Autodesk Inventor part; units mm, degrees
ref_plane "YZ Plane" through (0, 0, 0) normal (1, 0, 0) x (0, 1, 0)
ref_plane "XZ Plane" through (0, 0, 0) normal (0, 1, 0) x (-1, 0, 0)
ref_plane "XY Plane" through (0, 0, 0) normal (0, 0, 1) x (1, 0, 0)
sketch "Sketch1" plane through (0, 0, 0) normal (0, 1, 0) x (-1, 0, 0)
  line L0 (0, 0) -> (38.1, 0)
  line L1 (38.1, 0) -> (38.1, -50.8)
  line L2 (38.1, -50.8) -> (0, -50.8)
  line L3 (0, -50.8) -> (0, 0)
  line L4 (38.1, -50.8) -> (33.02, -50.8)
  line L5 (33.02, -50.8) -> (33.02, 0)
  line L6 (33.02, 0) -> (38.1, 0)
  line L7 (38.1, 0) -> (38.1, -50.8)
  line L8 (0, -50.8) -> (5.08, -50.8)
  line L9 (5.08, -50.8) -> (5.08, 0)
  line L10 (5.08, 0) -> (0, 0)
  line L11 (0, 0) -> (0, -50.8)
  dimension "d0" = 38.1
  dimension "d1" = 50.8
  dimension "d2" = 5.08
  dimension "d3" = 5.08
extrude "Extrusion1" add sketch "Sketch1" along normal blind 25.4 contours L0 L9 L2 L3 | L0 L1 L2 L5
extrude "Extrusion2" add sketch "Sketch1" against normal blind 13.97
sketch "Sketch2" plane through (0, 25.4, 0) normal (1, 0, 0) x (0, 0, -1)
  line L0 (50.8, 0) -> (0, 0)
  line L1 (25.4, 0) -> (25.4, -12.7)
  point P0 (0, -25.4)
  dimension "d8" = 12.7
hole "Hole1" at (0, 12.7, -25.4) direction (-1, 0, 0) diameter 6.7564 end through all
sketch "Sketch3" plane through (0, -13.97, 0) normal (0, -1, 0) x (1, 0, 0)
  line L0 (-38.1, -28.7782) -> (-38.1, -22.0218)
  line L1 (-38.1, -25.4) -> (-19.05, -25.4)
  line L2 (0, 0) -> (-38.1, 0)
  line L3 (-14.605, -50.8) -> (-23.495, -50.8)
  line L4 (-23.495, -50.8) -> (-23.495, 0)
  line L5 (-23.495, 0) -> (-14.605, 0)
  line L6 (-14.605, 0) -> (-14.605, -50.8)
  line L7 (-14.605, -50.8) -> (-23.495, 0) construction
  line L8 (-23.495, -50.8) -> (-14.605, 0) construction
  circle A0 centre (-19.05, -25.4) radius 9.906
  line L9 (-38.1, -50.8) -> (0, -50.8)
  line L10 (0, -50.8) -> (0, 0)
  line L11 (0, 0) -> (-38.1, 0)
  line L12 (-38.1, 0) -> (-38.1, -50.8)
  line L13 (-38.1, -50.8) -> (0, 0) construction
  line L14 (0, -50.8) -> (-38.1, 0) construction
  point P0 (-14.605, -16.5473)
  point P1 (-14.605, -34.2527)
  point P2 (-23.495, -34.2527)
  point P3 (-23.495, -16.5473)
  dimension "d16" = 19.05
  dimension "d17" = 8.89
  dimension "d18" = 19.812
extrude "Extrusion3" add sketch "Sketch3" along normal blind 13.97 contours L0 L1 A0 L4 L9 L12 | L0 L12 L2 L4 A0 L1 | L6 A0 L2 L10 L9
fillet "Fillet1" radius 3.175 14 edges at (-38.1, -1.27, -50.8) (0, -1.27, -50.8) (-7.3025, -27.94, -50.8) (0, -27.94, -25.4) (-30.7975, -27.94, -50.8) (-7.3025, -27.94, 0) (-30.7975, -27.94, 0) (-38.1, -27.94, -25.4) (-38.1, -1.27, 0) (0, -1.27, 0) (-14.605, -27.94, -42.5264) (-14.605, -27.94, -8.2736) (-23.495, -27.94, -8.2736) (-23.495, -27.94, -42.5264)
fillet "Fillet2" radius 3.175 14 edges at (-19.05, -13.97, 0) (-19.05, -13.97, -50.8) (-24.4249, -27.0101, -0.9299) (-23.495, -19.3675, 0) (-13.6751, -27.0101, -0.9299) (-14.605, -19.3675, 0) (-13.6751, -27.0101, -49.8701) (-7.3025, -27.94, -47.625) (-3.175, -27.0101, -49.8701) (-14.605, -19.3675, -50.8) (-34.925, -27.0101, -49.8701) (-30.7975, -27.94, -47.625) (-24.4249, -27.0101, -49.8701) (-23.495, -19.3675, -50.8)
properties part number "Sample Holder end for 8020-valveholder"
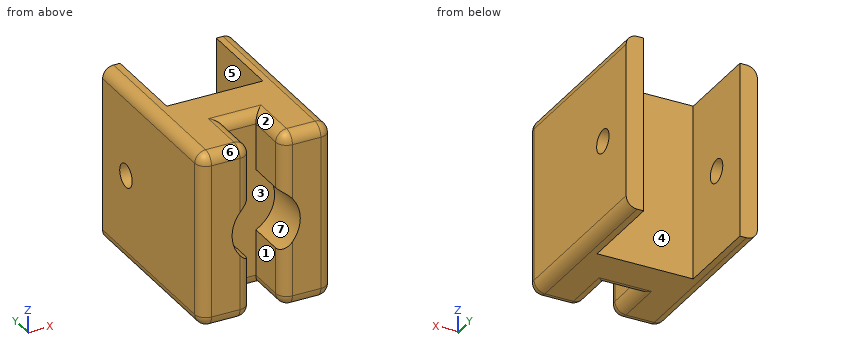
Source: CAD feature listing. Evaluate the final solid. Frame: model axes, mm. Face numbers are marked on the shaded views. A direction names the side the tool comes from. Give positions to 0.01 mm unless a question says otherwise; leave off trailing zeros. Write each loop counter-clockwise with the first axis right and the second up, starting at its lowest first coordinate (ties: lowest second). Pieces come first, ordered by that corner, then holes.
1. Pull-direction query (Z, two-part tool) for the marked faces 5, 6 and 7; classes: +Z half, -Z half, draft (parallel to the pull), parting line (faces both ways), or undercut.
2. Section query D-D (x = -7.5). Return the cut outline in (y, z) (3 decimals).
3. Access query for the marked faces 1, 2, 3 and 4. Directions: +Z, -Z, +X, -X, +Y, -Y. A direction counts if a zero-diameter tool reaches every point of the face in a straight line with its end or side. Return the directions, or none.
4. Section query C-C (y = 12.7). Return the cut outline in (x, z) (3 decimals), then the cut area to 3 significant figures.
5. Section query B-B (z = -25.4). Return the cut outline in (x, y) (3 decimals).
6. First-contact query: pin 1 (10 mm diameter, centred on x = -19.5, z = -25.5, fed in from -Y); pin 2 (8.5 mm diameter, centred on x = -13, z = -34, fed in from +Y). Flat tips, straight axial feed; report the tip coordinate or a pass-through.
7. Material intervals for line 1 along X through (y, z) = (18.5, -17); line 2 along X through (y, z) = (-16.5, -3); line 3 along Z through (x, y) = (-3.85, 12.7), sorted ascending.
8. Section query A-A (y = -16.5). Return the cut outline in (x, z) (3 decimals), then the cut area to 3 significant figures.
Output values:
1. face 5: draft
1. face 6: +Z half
1. face 7: undercut
2. outline: (-27.94, -47.625) arc R3.175 ccw to (-24.765, -50.8) - (0, -50.8) - (0, 0) - (-24.765, 0) arc R3.175 ccw to (-27.94, -3.175) - close
3. face 1: +Z, -Z, -Y
3. face 2: +Z, -Y
3. face 3: -Y
3. face 4: +Z, -Z, +Y
4. outline: (-38.1, -47.625) arc R3.175 ccw to (-34.925, -50.8) - (-33.02, -50.8) - (-33.02, -28.778) - (-38.1, -28.778) - close; (-38.1, -22.022) - (-33.02, -22.022) - (-33.02, 0) - (-34.925, 0) arc R3.175 ccw to (-38.1, -3.175) - close; (-5.08, -50.8) - (-3.175, -50.8) arc R3.175 ccw to (0, -47.625) - (0, -28.778) - (-5.08, -28.778) - close; (-5.08, -22.022) - (0, -22.022) - (0, -3.175) arc R3.175 ccw to (-3.175, 0) - (-5.08, 0) - close
4. area: 439 mm2
5. outline: (-38.1, -24.765) arc R3.175 ccw to (-34.925, -27.94) - (-28.956, -27.94) - (-28.956, -13.97) - (-9.144, -13.97) - (-9.144, -27.94) - (-3.175, -27.94) arc R3.175 ccw to (0, -24.765) - (0, 9.322) - (-5.08, 9.322) - (-5.08, 0) - (-33.02, 0) - (-33.02, 9.322) - (-38.1, 9.322) - close; (-38.1, 16.078) - (-33.02, 16.078) - (-33.02, 25.4) - (-38.1, 25.4) - close; (-5.08, 16.078) - (0, 16.078) - (0, 25.4) - (-5.08, 25.4) - close
6. pin 1: stops at y = -13.97
6. pin 2: stops at y = 0
7. line 1: x = -38.1 to -33.02, -5.08 to 0
7. line 2: x = -38.1 to -23.5, -14.6 to 0
7. line 3: z = -50.8 to -28.78, -22.02 to 0
8. outline: (-38.1, -47.625) arc R3.175 ccw to (-34.925, -50.8) - (-26.67, -50.8) arc R3.175 ccw to (-23.495, -47.625) - (-23.495, -34.253) arc R9.906 cw to (-23.495, -16.547) - (-23.495, -3.175) arc R3.175 ccw to (-26.67, 0) - (-34.925, 0) arc R3.175 ccw to (-38.1, -3.175) - close; (-14.605, -47.625) arc R3.175 ccw to (-11.43, -50.8) - (-3.175, -50.8) arc R3.175 ccw to (0, -47.625) - (0, -3.175) arc R3.175 ccw to (-3.175, 0) - (-11.43, 0) arc R3.175 ccw to (-14.605, -3.175) - (-14.605, -16.547) arc R9.906 cw to (-14.605, -34.253) - close
8. area: 1,330 mm2
